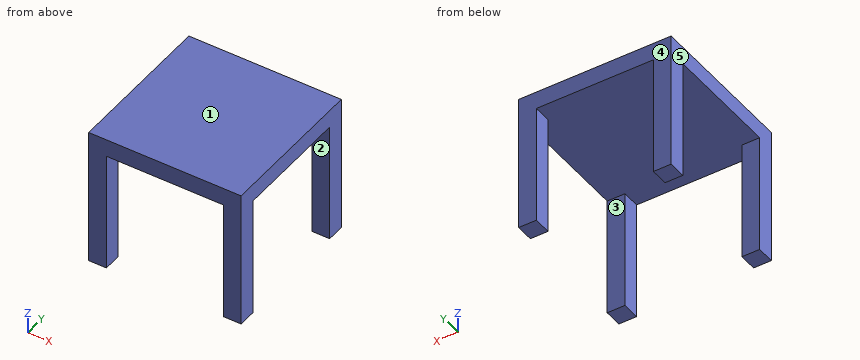
```python
from build123d import *

# Parameters (mm, degrees)
F1_W     = 430
F1_H     = 430
F2_DEPTH = 50
F3_W     = 50
F3_H     = 50
F4_DEPTH = 340


with BuildPart() as f2:
    # F1 (on offset) → F2 (new body)
    with BuildSketch(Plane.XY.offset(390)):
        Rectangle(F1_W, F1_H)
    extrude(amount=-F2_DEPTH)

    # F3 (on face) → F4 (join, through all)
    with BuildSketch(Plane(origin=(0, 0, 340), x_dir=(1, 0, 0), z_dir=(0, 0, -1))):
        with Locations((190, 190)):
            Rectangle(F3_W, F3_H)
        with Locations((-190, 190)):
            Rectangle(F3_W, F3_H)
        with Locations((-190, -190)):
            Rectangle(F3_W, F3_H)
        with Locations((190, -190)):
            Rectangle(F3_W, F3_H)
    extrude(amount=F4_DEPTH)


solid = f2.part
```
The listing builds one solid part. Answer for the finished solid, in the listing's coordinates (mm). Face numbers are marked on the shaded views. A direction names the side the tool comes from. Give positions to 0.01 mm unless a question says otherwise; leave off trailing zeros. Write each loop counter-clockwise with the first axis right and the second up, starting at its lowest first coordinate (ties: lowest second). Pieces come first, ordered by that corner, then holes. Notation, with made-up numbers: (87, 70) -> (142, 70) arc R17 ccw to (142, 88) -> close; hole circle Ø9 at (82.25, -8). An arc over 180 degrees is marked (long way). Write item = value, one per line. Start each with the question number.
1) Determine the mould class of the marked faces 3, 4 and 5 for opening direction Y: +Y half, -Y half, draft (parallel to the pull), parting line (faces both ways), or undercut.
2) The part is cut by section B-B, the plane y = -178. Determine the outline of the cut face in (x, z).
3) The part is cut by section A-A, the plane z = 242. Determine the outline of the cut face in (x, y), and give its area (3 significant figures).
4) Straight lines are drawn through the part: line 1 along X through (y, z) = (-174, 71.5); line 2 along Z through (x, y) = (-8, 38). For each, find the intervals that lie inside material, in ascending order.
5) This flat-tipped pin is pushed along its axis until it touches: pin 1 (12 mm diameter, centred on x = 151, y = -150, fed in from -Z). Where does it stop, or does it pass through?
6) Which of the six approach directions +Z, -Z, +X, -X, +Y, -Y give full straight-line access (tool end or side, diameter ignored) to the marked faces 1 and 2?
7) The part is cut by section D-D, the plane x = -109. Determine the outline of the cut face in (y, z), and give its area (3 significant figures).
Solutions:
q1.face_3 = undercut
q1.face_4 = +Y half
q1.face_5 = draft
q2.outline = (-215, 0) -> (-165, 0) -> (-165, 340) -> (165, 340) -> (165, 0) -> (215, 0) -> (215, 390) -> (-215, 390) -> close
q3.outline = (-215, -215) -> (-165, -215) -> (-165, -165) -> (-215, -165) -> close; (-215, 165) -> (-165, 165) -> (-165, 215) -> (-215, 215) -> close; (165, -215) -> (215, -215) -> (215, -165) -> (165, -165) -> close; (165, 165) -> (215, 165) -> (215, 215) -> (165, 215) -> close
q3.area = 10,000 mm²
q4.line_1 = -215 to -165, 165 to 215
q4.line_2 = 340 to 390
q5.pin_1 = 340
q6.face_1 = +Z, +X, -X, +Y, -Y
q6.face_2 = -Z, +X, -X
q7.outline = (-215, 340) -> (215, 340) -> (215, 390) -> (-215, 390) -> close
q7.area = 21,500 mm²
